Part model, mm, in its own coordinate system. A direction names the side the tool comes from. Round coordinates to 2 decimals unless told otherwise and drop trailing zeros. Order: outer loops, then holes, each group sorted by start corner. A loop starts at its lowest first (then second) coordinate and runs counter-clockwise, first axis right, second up. Notation, with made-up numbers: M 84.25,57 L 143.25,57 A21 cw 143.25,65 Z; hole C 28.25,-3 d4. An arc over 180 degrees is marked long. Write each question's results on one line, items separated by ' | '. Start each with the question number.
1. Band-saw the part on B-B, the plane x = 3. List the corners of the cut face in (y, z), then the cut area to 3 significant figures.
2. Probe L1, parallel to X at y = -10, z = 3.2; L2, parallel to Z at x = -2.25, y = -11.75; L3, parallel to Y at x = 0, z = 7.5. List the from-to ranges inside material, lowest first. Write a range as [from, to].
3. Which spindle directions (+Z, -Z, +X, -X, +Y, -Y) get a long thin tool onto all of the face, cutting with end or side? Do faces 1 (the face through (4.64, 0.13, 6.14)), 2 (the face through (0.165, 6.254, 8.298)). Say none if no direction does.
4. Drop flat-ended pins along their axis: pin 1 Ø1.5 at (x, y) = (-3.5, 2.5) entering from +Z; pin 2 Ø3.5 at (x, y) = (0, 10) entering from +Z; pin 3 Ø4 at (x, y) = (1, 9.5) entering from +Z; pin 4 Ø6 at (x, y) = (2, 8) entering from +Z. Give the stop position or say it passes through.
5. Band-saw the part on A-A, the plane y = 0. List the corners of the cut face in (x, z).
Autodesk Inventor part; units mm, degrees
ref_plane "1_2_XY" through (0, 0, 0) normal (0, 0, 1) x (1, 0, 0)
ref_plane "1_2_YZ" through (0, 0, 0) normal (1, 0, 0) x (0, 1, 0)
ref_plane "1_2_ZX" through (0, 0, 0) normal (0, 1, 0) x (0, 0, 1)
sketch "Sketch_1" plane through (0, 0, 0) normal (0, 0, 1) x (1, 0, 0)
  line L0 (5, 0) -> (-5, 0)
  line L1 (-5, 14.5) -> (-5, 6.5)
  line L2 (-5, 6.5) -> (-4.5, 6)
  line L3 (-4.5, 6) -> (4.5, 6)
  line L4 (4.5, 6) -> (5, 6.5)
  line L5 (5, 6.5) -> (5, 14.5)
  line L6 (5, 14.5) -> (4.5, 15)
  line L7 (4.5, 15) -> (-4.5, 15)
  line L8 (-4.5, 15) -> (-5, 14.5)
revolve "Revolution1" add sketch "Sketch_1" angle 180 about axis through (5, 0, 0) along (1, 0, 0)
sketch "Sketch_2" plane through (0, 0, 0) normal (1, 0, 0) x (0, 1, 0)
  line L0 (-15, 0.75) -> (-15, -0.75)
  line L1 (-15, -0.75) -> (15, -0.75)
  line L2 (15, -0.75) -> (15, 0.75)
  line L3 (15, 0.75) -> (-15, 0.75)
extrude "Extrusion1" cut sketch "Sketch_2" along normal mid plane 10
sketch "Sketch_3" plane through (0, 0, 0) normal (1, 0, 0) x (0, 1, 0)
  line L0 (-10, 0) -> (-10, 15)
  line L1 (-10, 15) -> (-6.25, 15)
  line L2 (-6.25, 15) -> (-6.25, 5)
  line L3 (-6.25, 5) -> (-7.75, 5)
  line L4 (-7.75, 5) -> (-7.75, 0)
  line L5 (-7.75, 0) -> (-10, 0)
  line L6 (-10, 0) -> (-10, 15)
revolve "Revolution2" cut sketch "Sketch_3" angle 360 about axis through (0, -10, 0) along (0, 0, -1)
sketch "Sketch_4" plane through (0, 0, 0) normal (1, 0, 0) x (0, 1, 0)
  line L0 (10, 0) -> (10, 15)
  line L1 (10, 15) -> (13.75, 15)
  line L2 (13.75, 15) -> (13.75, 5)
  line L3 (13.75, 5) -> (12.25, 5)
  line L4 (12.25, 5) -> (12.25, 0)
  line L5 (12.25, 0) -> (10, 0)
  line L6 (10, 0) -> (10, 15)
revolve "Revolution3" cut sketch "Sketch_4" angle 360 about axis through (0, 10, 0) along (0, 0, -1)
ref_plane "1_2_XY" through (0, 0, 0) normal (0, 0, 1) x (1, 0, 0)
ref_plane "1_2_YZ" through (0, 0, 0) normal (1, 0, 0) x (0, 1, 0)
ref_plane "1_2_ZX" through (0, 0, 0) normal (0, 1, 0) x (0, 0, 1)
ref_plane "body_screw_XY" through (0, -10, 5) normal (0, 0, 1) x (1, 0, 0)
ref_plane "body_screw_YZ" through (0, -10, 5) normal (1, 0, 0) x (0, 1, 0)
ref_plane "body_screw_ZX" through (0, -10, 5) normal (0, 1, 0) x (0, 0, 1)
ref_plane "body_screw2_XY" through (0, 10, 5) normal (0, 0, 1) x (1, 0, 0)
ref_plane "body_screw2_YZ" through (0, 10, 5) normal (1, 0, 0) x (0, 1, 0)
ref_plane "body_screw2_ZX" through (0, 10, 5) normal (0, 1, 0) x (0, 0, 1)
properties part number "SSCSP12-10b"
Solution:
1) outline: M -14.98,0.75 L -5.95,0.75 A6 cw 5.95,0.75 L 14.98,0.75 A15 ccw 12.25,8.66 L 12.25,5 L 7.75,5 L 7.75,12.84 A15 ccw -7.75,12.84 L -7.75,5 L -12.25,5 L -12.25,8.66 A15 ccw Z | area: 229 mm^2
2) L1: [-5, -2.25], [2.25, 5] | L2: [0.75, 5] | L3: [-6.25, 6.25]
3) face 1: -Z, +X | face 2: +Z
4) pin 1: z = 14.9 | pin 2: through | pin 3: z = 5 | pin 4: z = 14.14
5) outline: M -5,6.5 L -4.5,6 L 4.5,6 L 5,6.5 L 5,14.5 L 4.5,15 L -4.5,15 L -5,14.5 Z
